Here's how the part is built. I have some questions about the finished solid (model axes, mm). Round coordinates to 2 decimals unless told otherwise and drop trailing zeros. Loops run counter-clockwise (first coordinate to the right, second up) from the corner with the lowest first, then second, coordinate; pieces in that order, holes last. Notation, with made-up numbers: M -24,56 L -14,56 A31 ccw -14,93 Z; hole C 15,-23.75 d3. An arc over 180 degrees is marked long. Write item = value, one per line. Start each with the question number.
from build123d import *

# Parameters (mm, degrees)
CROQUIS1_W              = 105
CROQUIS1_H              = 150
SALIENTE_EXTRUIR1_DEPTH = 10
CROQUIS2_R              = 2.25
CORTAR_EXTRUIR1_DEPTH   = 93.093702282
CROQUIS3_R              = 2.25
CORTAR_EXTRUIR2_DEPTH   = 93.093702282


with BuildPart() as part:
    # Croquis1 → Saliente-Extruir1 (new body)
    with BuildSketch(Plane(origin=(0, 0, 0), x_dir=(0, 0, -1), z_dir=(1, 0, 0))):
        Rectangle(CROQUIS1_W, CROQUIS1_H)
    extrude(amount=SALIENTE_EXTRUIR1_DEPTH)

    # Croquis2 → Cortar-Extruir1 (cut, through all)
    with BuildSketch(Plane(origin=(10, 0, 0), x_dir=(0, 0, -1), z_dir=(1, 0, 0))):
        with Locations((-42.5, 70)):
            Circle(CROQUIS2_R)
        with Locations((0, 70)):
            Circle(CROQUIS2_R)
        with Locations((42.5, 70)):
            Circle(CROQUIS2_R)
    extrude(amount=-CORTAR_EXTRUIR1_DEPTH, mode=Mode.SUBTRACT)

    # Croquis3 → Cortar-Extruir2 (cut, through all)
    with BuildSketch(Plane(origin=(10, 0, 0), x_dir=(0, 0, -1), z_dir=(1, 0, 0))):
        with Locations((25, 30)):
            Circle(CROQUIS3_R)
        with Locations((-25, 30)):
            Circle(CROQUIS3_R)
        with Locations((25, -55)):
            Circle(CROQUIS3_R)
        with Locations((-25, -55)):
            Circle(CROQUIS3_R)
    extrude(amount=-CORTAR_EXTRUIR2_DEPTH, mode=Mode.SUBTRACT)


solid = part.part
Item 1: I want a section at C-C, the plane y = 70. List the corners of the cut face in (x, z) for me, then the cut area to 3 significant figures.
Item 2: Please list where these lines run through material, in increasing order: line 1 (Y direction, x = 3.25, z = -42.5); line 2 (Y direction, x = 8.75, z = 27); line 3 (Y direction, x = 3, z = 1). Write a range as [from, to].
Item 3: I want a section at B-B, the plane z = 25. List the corners of the cut face in (x, y) for me.
Item 4: We'd pull the mould along Z, two halves only. Please class faces 1 (the cylindrical face through (5.07, -53.103, 23.79)), 2 (the flat face through (10, 1, 1)), 3 (the flat face through (5, -1, -52.5)): released by +Z, released by -Z, zero draft, split by the parting line, or undercut.
Item 5: I want a section at D-D, the plane z = 42.5. List the corners of the cut face in (x, y) for me.
Item 6: Will this pin go through, and if not, where does the flat tip stop? pin 1 Ø3.5 at (y, z) = (-55, 25) entering from -X.
Item 7: I want a section at A-A, the plane y = -55. List the corners of the cut face in (x, z) for me, then the cut area to 3 significant figures.
Worked out:
q1.outline = M 0,-52.5 L 10,-52.5 L 10,-44.75 L 0,-44.75 Z; M 0,-40.25 L 10,-40.25 L 10,-2.25 L 0,-2.25 Z; M 0,2.25 L 10,2.25 L 10,40.25 L 0,40.25 Z; M 0,44.75 L 10,44.75 L 10,52.5 L 0,52.5 Z
q1.area = 915 mm2
q2.line_1 = [-75, 67.75], [72.25, 75]
q2.line_2 = [-75, -56.03], [-53.97, 28.97], [31.03, 75]
q2.line_3 = [-75, 67.98], [72.02, 75]
q3.outline = M 0,-75 L 10,-75 L 10,-57.25 L 0,-57.25 Z; M 0,-52.75 L 10,-52.75 L 10,27.75 L 0,27.75 Z; M 0,32.25 L 10,32.25 L 10,75 L 0,75 Z
q4.face_1 = undercut
q4.face_2 = zero draft
q4.face_3 = released by -Z
q5.outline = M 0,-75 L 10,-75 L 10,67.75 L 0,67.75 Z; M 0,72.25 L 10,72.25 L 10,75 L 0,75 Z
q6.pin_1 = through
q7.outline = M 0,-52.5 L 10,-52.5 L 10,-27.25 L 0,-27.25 Z; M 0,-22.75 L 10,-22.75 L 10,22.75 L 0,22.75 Z; M 0,27.25 L 10,27.25 L 10,52.5 L 0,52.5 Z
q7.area = 960 mm2
